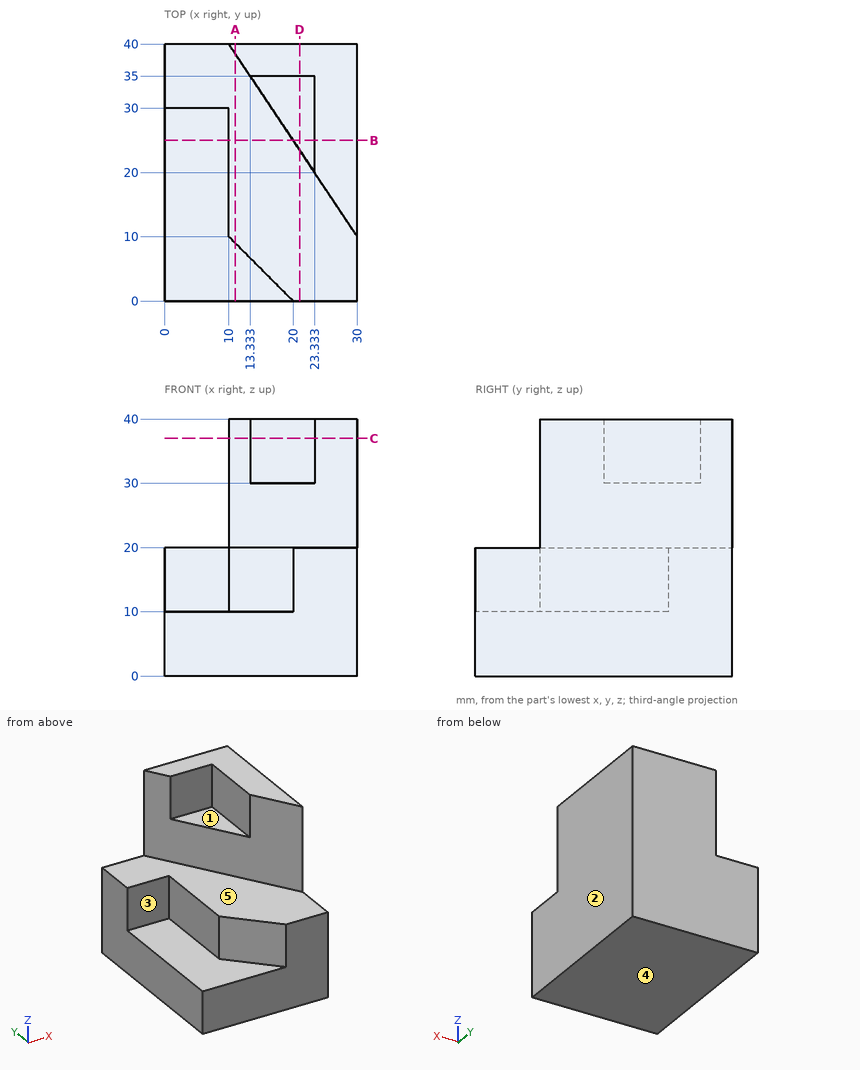
Drawing for the job (mm, zero at the part's lowest x, y, z). A direction names the side the tool comes from. Give positions to 0.01 mm unless a question says otherwise; leave off trailing zeros. Loops run counter-clockwise (first coordinate to the right, second up) from the corner with the lowest first, then second, coordinate; pieces in that order, holes last.
(1) Band-saw the part on D-D (x = 21). Write the cut outline in (y, z).
Return value:
outline: (0, 0) - (40, 0) - (40, 40) - (35, 40) - (35, 30) - (23.5, 30) - (23.5, 20) - (0, 20) - close
(2) 3-axis set-ups, long thin cutter, end or side, ignore diameter. For the marked faces 1 and 2: which of +Z, -Z, +X, -X, +Y, -Y reach the whole face in a straight line?
Return value:
face 1: +Z, -X, -Y
face 2: +Z, -Z, +X, +Y, -Y
(3) Band-saw the part on A-A (x = 11). Write the cut outline in (y, z).
Return value:
outline: (0, 0) - (40, 0) - (40, 40) - (38.5, 40) - (38.5, 20) - (9, 20) - (9, 10) - (0, 10) - close
(4) Band-saw the part on B-B (y = 25). Write the cut outline in (x, z), and give its area (3 significant figures).
Return value:
outline: (0, 0) - (30, 0) - (30, 40) - (23.33, 40) - (23.33, 30) - (20, 30) - (20, 20) - (10, 20) - (10, 10) - (0, 10) - close
area: 667 mm2
(5) Pull direction Z, two halves, no side cores. Call the marked faces 3, 4 and 5: pulls with the +Z half, pulls with the -Z half, needs draft (parallel to the pull), parting line crosses it, or undercut.
Return value:
face 3: needs draft
face 4: pulls with the -Z half
face 5: pulls with the +Z half
(6) Pin check, flat tips, straight feed: pin 1 (3 mm diameter, centred on y = 26.5, z = 33, fed in from -X); pin 2 (4 mm diameter, centred on y = 11.5, z = 27, fed in from -X); pin 3 (3 mm diameter, centred on x = 16, y = 30, fed in from +Z); pin 4 (11 mm diameter, centred on x = 2.5, z = 13, fed in from -Y). Stop position of each tip, or through.
Return value:
pin 1: stops at x = 23.33
pin 2: stops at x = 27.67
pin 3: stops at z = 30
pin 4: stops at y = 0
(7) Band-saw the part on C-C (z = 37). Write the cut outline in (x, y).
Return value:
outline: (10, 40) - (13.33, 35) - (23.33, 35) - (23.33, 20) - (30, 10) - (30, 40) - close
(8) Drill centre lines: line 1 along Z through (x, y) = (10, 2); line 2 along Y through (x, z) = (7, 15); line 3 along Z through (x, y) = (12.5, 20). Where is each one in solid material? Low to high.
Return value:
line 1: z = 0 to 10
line 2: y = 30 to 40
line 3: z = 0 to 20
